The drawing under review shows one solid part. Ordinate dimensions are in mm from its lowest x, y, z. A direction names the side the tool comes from. Give positions to 0.01 mm unless a question says otherwise; leave off trailing zeros. Order: outer loops, then holes, each group sorted by start corner. A loop starts at its lowest first (then second) coordinate and runs counter-clockwise, first axis right, second up. Notation, with made-up numbers: (-3, -30) -> (5, -30) arc R22 ccw to (5, -13) -> close; hole circle Ø4 at (-19.75, -4). An arc over 180 degrees is marked (long way). Use CSV: the item, a comma, the result in double quotes. Start each with the question number.
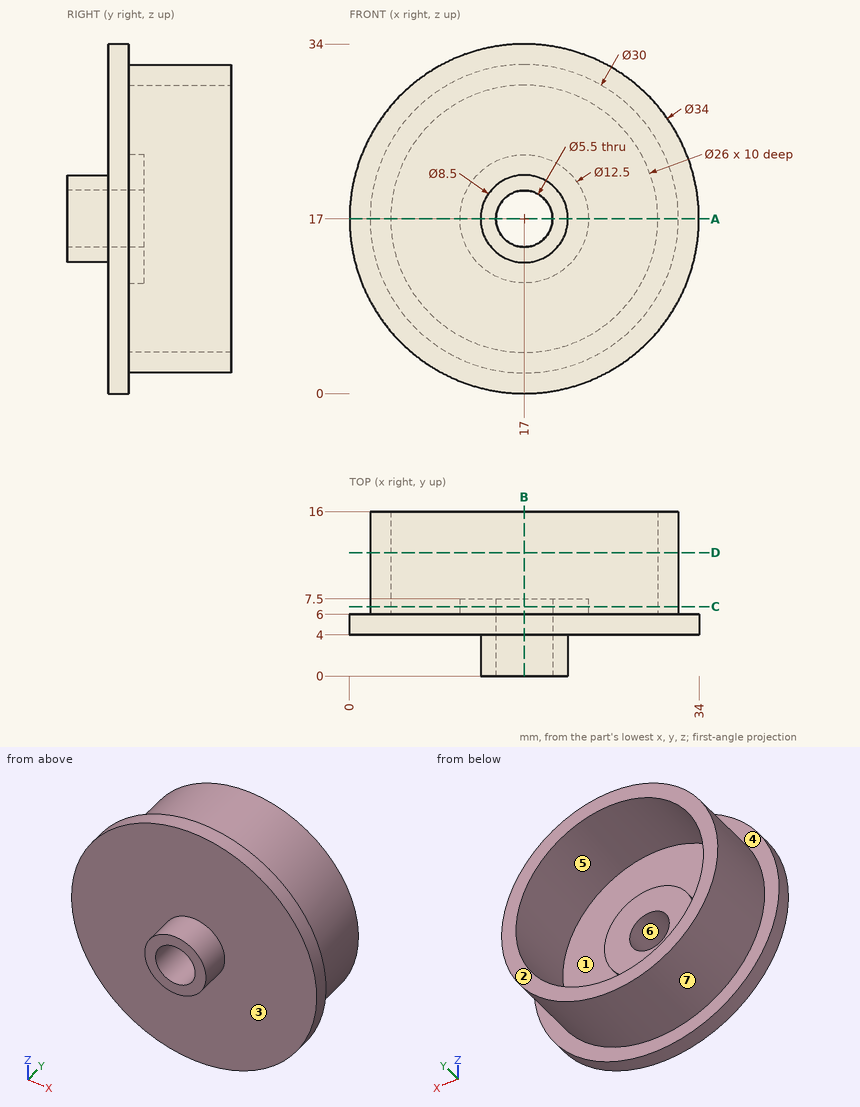
1. Consider section B-B (x = 17). State the section outline as (y, z) points, plus the area to 4 significant figures.
2. Clearance check with flat-ended pins moving along their axes: P1, Ø8, axis at x = 17.5, y = 14, coming from the -Z side; P2, Ø10, axis at x = 18.5, z = 16.5, coming from the +Y side; P3, Ø8, axis at x = 15.5, y = 12.5, coming from the +Z side. State where each tip first meets the part, or that it passes through.
3. To check wall thickness, follow L1, parallel to Z at x = 17, y = 8.25; L2, parallel to X at y = 5.75, z = 17. State the ranges of each line that lie inside material, in increasing order. Write a range as [from, to].
4. For the marked faces 1, 2 and 3, list the 3-axis set-ups (+Z, -Z, +X, -X, +Y, -Y) from which the entire face can be reached by the end or side of a thin tool; tool diameter is ignored.
5. Consider section C-C (y = 6.75). State the section outline as (x, z) points, plus the area to 3 significant figures.
6. Consider section A-A (z = 17). State the section outline as (x, y) points.
7. Consider section D-D (y = 12). State the section outline as (x, z) points, plus the area to 3 significant figures.
8. Draft analysis for pull direction Z (two halves, no side actions). For the marked faces 4, 5, 6 and 7, state which applies: +Z half, -Z half, draft (parallel to the pull), parting line (faces both ways), or undercut.
Answer list:
1,outline,"(0, 12.75) -> (4, 12.75) -> (4, 0) -> (6, 0) -> (6, 2) -> (16, 2) -> (16, 4) -> (6, 4) -> (6, 10.75) -> (7.5, 10.75) -> (7.5, 14.25) -> (0, 14.25) -> close; (0, 19.75) -> (7.5, 19.75) -> (7.5, 23.25) -> (6, 23.25) -> (6, 30) -> (16, 30) -> (16, 32) -> (6, 32) -> (6, 34) -> (4, 34) -> (4, 21.25) -> (0, 21.25) -> close"
1,area,"119.5 mm2"
2,P1,"z = 2"
2,P2,"y = 7.5"
2,P3,"z = 32"
3,L1,"[2, 4], [30, 32]"
3,L2,"[0, 14.25], [19.75, 34]"
4,face 1,"+Y"
4,face 2,"+Z, -Z, +X, -X, +Y"
4,face 3,"-Y"
5,outline,"circle Ø30 at (17, 17); circle Ø12.5 at (17, 17); hole circle Ø26 at (17, 17); hole circle Ø5.5 at (17, 17)"
5,area,"275 mm2"
6,outline,"(0, 4) -> (12.75, 4) -> (12.75, 0) -> (14.25, 0) -> (14.25, 7.5) -> (10.75, 7.5) -> (10.75, 6) -> (4, 6) -> (4, 16) -> (2, 16) -> (2, 6) -> (0, 6) -> close; (19.75, 0) -> (21.25, 0) -> (21.25, 4) -> (34, 4) -> (34, 6) -> (32, 6) -> (32, 16) -> (30, 16) -> (30, 6) -> (23.25, 6) -> (23.25, 7.5) -> (19.75, 7.5) -> close"
7,outline,"circle Ø30 at (17, 17); hole circle Ø26 at (17, 17)"
7,area,"176 mm2"
8,face 4,"draft"
8,face 5,"undercut"
8,face 6,"undercut"
8,face 7,"parting line"
